```python
from build123d import *

# Parameters (mm, degrees)
F0_W     = 990.6
F0_H     = 585.7875
F1_DEPTH = 2.5
F2_W     = 690.6
F2_H     = 25
F3_DEPTH = 0.5


with BuildPart() as f1:
    # F0 (on Front) → F1 (new body)
    with BuildSketch(Plane.XZ):
        Rectangle(F0_W, F0_H)
    extrude(amount=F1_DEPTH)

    # F2 (on face) → F3 (join)
    with BuildSketch(Plane.XZ.offset(2.5)):
        with Locations((-5, -305.39375)):
            Rectangle(F2_W, F2_H)
    extrude(amount=-F3_DEPTH)


solid = f1.part
```
Can you work these out from the model? Positions are in its coordinate system, mm. A direction names the side the tool comes from. Round coordinates to 2 decimals unless told otherwise and drop trailing zeros. Loops run counter-clockwise (first coordinate to the right, second up) from the corner with the lowest first, then second, coordinate; pieces in that order, holes last. Notation, with made-up numbers: M 39,79.25 L 91,79.25 A18 ccw 91,84.25 Z; hole C 8.5,23.5 d9. An arc over 180 degrees is marked long. Write item = value, one per line. Start each with the question number.
(1) Which directions (+Z, -Z, +X, -X, +Y, -Y) give clear straight access to the entire face, cutting with the end or side of a thin tool? Please do faces 1 (the face through (-7, 0, 4)), 2 (the face through (-10, -2, -305)).
(2) Suppose I cut it at A-A on x = 422.5. Write out the boundary of the cut face in (y, z), plus the area to 3 significant figures.
(3) Suppose I cut it at C-C on x = 102.5. Write out the boundary of the cut face in (y, z).
(4) Suppose I cut it at B-B on y = -1.4. Write out the boundary of the cut face in (x, z).
(5) I'm going to push flat-ended pins straight in: P1, Ø6, axis at x = -56.5, z = -28, coming from the +Y side; P2, Ø0.6, axis at y = -2, z = -301, coming from the -X side; P3, Ø7.5, axis at x = -82, z = -301, coming from the +Y side; P4, Ø0.8, axis at x = -103, y = -1.5, coming from the -Z side. Where does each tip first touch, or does it pass through?
(6) I need wall thicknesses on line 1 along Z through (x, y) = (-353.5, -0.8). Which ranges of the line are inside material? Lowest first, please.
Answer block:
q1.face_1 = +Z, -Z, +X, -X, +Y
q1.face_2 = -Z, +X, -X, +Y
q2.outline = M -2.5,-292.89 L 0,-292.89 L 0,292.89 L -2.5,292.89 Z
q2.area = 1,460 mm²
q3.outline = M -2.5,-317.89 L -2,-317.89 L -2,-292.89 L 0,-292.89 L 0,292.89 L -2.5,292.89 Z
q4.outline = M -495.3,-292.89 L 495.3,-292.89 L 495.3,292.89 L -495.3,292.89 Z
q5.P1 = 0
q5.P2 = -350.3
q5.P3 = -2
q5.P4 = -292.89
q6.line_1 = -292.89 to 292.89
